Autodesk Inventor part; units mm, degrees
ref_plane "YZ Plane" through (0, 0, 0) normal (1, 0, 0) x (0, 1, 0)
ref_plane "XZ Plane" through (0, 0, 0) normal (0, 1, 0) x (-1, 0, 0)
ref_plane "XY Plane" through (0, 0, 0) normal (0, 0, 1) x (1, 0, 0)
sketch "Esquisse1" plane through (0, 0, 0) normal (0, 0, 1) x (1, 0, 0)
  circle A0 centre (-41.5, 69.6) radius 12.5
  circle A1 centre (-41.5, 69.6) radius 11
  circle A2 centre (-41.5, 69.6) radius 13
  point P0 (0, 0)
  dimension "d11" = 0.5
  dimension "d15" = 2
ref_plane "Plan de construction2" through (-41.5, 69.6, 0) normal (0, -1, 0) x (0, 0, 1)
ref_plane "Plan de construction1" through (0, 0, -152.2) normal (0, -1, 0) x (0, 0, 1)
sketch "Esquisse2" plane through (-41.5, 69.6, 0) normal (0, -1, 0) x (0, 0, 1)
  point P0 (0, -41.5)
  point P1 (0, 0)
  point P2 (-5, 0)
  dimension "d1" = 5
ref_plane "Plan de construction4" through (-41.5, 69.6, -5) normal (0, 0, 1) x (1, 0, 0)
ref_plane "Plan de construction3" through (0, 0, 0) normal (0, 0, 1) x (1, 0, 0)
sketch "Esquisse3" plane through (-41.5, 69.6, -5) normal (0, 0, 1) x (1, 0, 0)
  circle A0 centre (0, 0) radius 12.5
  circle A1 centre (0, 0) radius 9.5
  circle A2 centre (0, 0) radius 11.5
  point P0 (41.5, -69.6)
  dimension "d13" = 2
  dimension "d14" = 1
ref_plane "Plan de construction5" through (-41.5, 69.6, 0) normal (0, 0, 1) x (1, 0, 0)
loft "Lissage2" add profiles "Esquisse3", "Esquisse1" contours A1 | A2 / A0 | A1 | A2
sketch "Esquisse5" plane through (-41.5, 69.6, 0) normal (0, 0, 1) x (1, 0, 0)
  circle A0 centre (0.1842, -0.128) radius 10.7757
  circle A1 centre (0, 0) radius 13
  point P0 (41.5, -69.6)
  dimension "d20" = 2
extrude "Extrusion2" cut sketch "Esquisse5" against normal blind 10 contours A0
ref_plane "Plan de construction6" through (0, 0, 0) normal (-1, 0, 0) x (0, -1, 0)
sketch "Esquisse6" plane through (0, 0, 0) normal (-1, 0, 0) x (0, -1, 0)
  point P0 (0, 0)
sketch "Esquisse7" plane through (-41.5, 69.6, 0) normal (0, 0, 1) x (1, 0, 0)
  circle A0 centre (0.1842, -0.128) radius 10.7757
  circle A1 centre (0, 0) radius 13
  point P0 (41.5, -69.6)
sketch "Esquisse8" plane through (0, 0, 0) normal (-1, 0, 0) x (0, -1, 0)
  line L0 (0, 5) -> (-101.6415, 5)
  point P0 (0, 0)
  dimension "d23" = 5
revolve "Révolution1" add sketch "Esquisse7" angle 90 about axis through (0, 0, 5) along (0, 1, 0)
sketch "Esquisse9" plane through (-5, 69.6, 46.5) normal (1, 0, 0) x (0, 0, -1)
  circle A0 centre (0, 0) radius 13
  circle A1 centre (0.1842, -0.128) radius 10.7757
  point P0 (46.5, -69.6)
  point P1 (13, 0)
  point P2 (10.9599, -0.128)
extrude "Extrusion3" add sketch "Esquisse9" along normal up to surface (5 mm away)
sketch "Esquisse10" plane through (0, 69.6, 46.5) normal (1, 0, 0) x (0, 0, -1)
  circle A0 centre (0.1842, -0.128) radius 10.7757
  line L0 (2.1644, -3.5577) -> (-1.7959, -3.5577)
  line L1 (-1.7959, -3.5577) -> (-3.7761, -0.128)
  line L2 (-3.7761, -0.128) -> (-1.7959, 3.3017)
  line L3 (-1.7959, 3.3017) -> (2.1644, 3.3017)
  line L4 (2.1644, 3.3017) -> (4.1445, -0.128)
  line L5 (4.1445, -0.128) -> (2.1644, -3.5577)
  line L6 (2.4473, -3.0677) -> (6.2069, -9.0635)
  line L7 (1.5742, -3.5577) -> (5.3525, -9.5834)
  line L8 (3.8616, 0.362) -> (10.9339, 0.62)
  line L9 (3.8494, -0.6391) -> (10.9569, -0.3798)
  line L10 (1.5986, 3.3017) -> (4.9112, 9.5555)
  line L11 (2.4595, 2.7906) -> (5.7886, 9.0755)
  line L12 (-2.0788, 2.8117) -> (-5.8384, 8.8074)
  line L13 (-1.2058, 3.3017) -> (-4.9841, 9.3273)
  line L14 (-3.4932, -0.618) -> (-10.5654, -0.8761)
  line L15 (-3.481, 0.3831) -> (-10.5885, 0.1237)
  line L16 (-1.2301, -3.5577) -> (-4.5428, -9.8115)
  line L17 (-2.091, -3.0466) -> (-5.4202, -9.3316)
  point P0 (46.5, -69.6)
  point P1 (3.8494, -0.6391)
  point P2 (10.9569, -0.3798)
  point P3 (10.9339, 0.62)
  point P4 (3.8616, 0.362)
  point P5 (2.4595, 2.7906)
  point P6 (5.7886, 9.0755)
  point P7 (4.9112, 9.5555)
  point P8 (1.5986, 3.3017)
  point P9 (-1.2058, 3.3017)
  point P10 (-4.9841, 9.3273)
  point P11 (-5.8384, 8.8074)
  point P12 (-2.0788, 2.8117)
  point P13 (-3.481, 0.3831)
  point P14 (-10.5885, 0.1237)
  point P15 (-10.5654, -0.8761)
  point P16 (-3.4932, -0.618)
  point P17 (-2.091, -3.0466)
  point P18 (-5.4202, -9.3316)
  point P19 (-4.5428, -9.8115)
  point P20 (-1.2301, -3.5577)
  dimension "d28" = 0.5
  dimension "d29" = 0.5
  dimension "d32" = 360
extrude "Extrusion4" add sketch "Esquisse10" against normal blind 2 contours A0 L9 L5 L4 L8 | L11 L4 L3 L10 A0 | L4 L5 L0 L1 L2 L3 | A0 L7 L0 L5 L6 | L13 L3 L2 L12 A0 | A0 L17 L1 L0 L16 | L15 L2 L1 L14 A0
properties part number "Aeration"
The listing builds one solid part. Answer for the finished solid, in the listing's coordinates (mm). A direction names the side the tool comes from. Round coordinates to 2 decimals unless told otherwise and drop trailing zeros. Write each question's results on one line, items separated by ' | '. Start each with the question number.
(1) For faces 1 (the flat face through (0, 70, 47)), 2 (the flat face through (-0.986, 75.872, 49.569)), determine the directions among +Z, -Z, +X, -X, +Y, -Y from which every point of the face is accessible in a straight line to the end or side of a thin tool.
(2) Each of these flat-tipped pins is pushed along its axis until it touches: P1, Ø1, axis at x = -29, y = 79, coming from the +Z side; P2, Ø12, axis at x = -29, y = 75.5, coming from the -Z side; P3, Ø1, axis at x = -26, y = 67.5, coming from the +Z side; P4, Ø12, axis at y = 76, z = 50, coming from the -X side. Where does it stop, or does it pass through?
(3) Find the intervals of material crossed by line 1 (Y direction, x = -8.5, z = 46); line 2 (X direction, y = 66, z = 22.5); line 3 (Z direction, x = -6.5, y = 60.5), in increasing order.
(4) Determine the mould class of faces 3 (the cylindrical face through (-35.523, 78.558, -2.465)), 4 (the flat face through (-0.99, 70.09, 39.15)), 5 (the cylindrical face through (-2.535, 69.028, 59.487)), 6 (the cylindrical face through (-2.54, 79.03, 41.34)) for opening direction Z: +Z half, -Z half, draft (parallel to the pull), parting line (faces both ways), or undercut.
Worked answers:
1) face 1: +Z, -Z, +X, +Y, -Y | face 2: +X
2) P1: stops at z = 47.31 | P2: stops at z = -5 | P3: stops at z = 53.25 | P4: stops at x = -36.97
3) line 1: y = 56.6 to 58.7, 80.24 to 82.6 | line 2: x = -51.32 to -48.71, -26.21 to -23.67 | line 3: z = 36.95 to 40.1, 52.1 to 55.61
4) face 3: draft | face 4: undercut | face 5: parting line | face 6: undercut
